Verification items for the finished model (mm, model axes). A direction names the side the tool comes from. Coordinates: 2 decimals unless noted, no trailing zeros. Order: outer loops, then holes, each group sorted by start corner. A loop starts at its lowest first (then second) coordinate and runs counter-clockwise, first axis right, second up. Notation, with made-up numbers: M 34,34.5 L 57,34.5 A17 ccw 57,56.5 Z; hole C 19.25,35.5 d2. An arc over 180 degrees is marked long. Return JSON: item names as keys, results as strings.
```python
from build123d import *

# Parameters (mm, degrees)
SKETCH1_W               = 89.5
SKETCH1_H               = 45.5
BOSS_EXTRUDE1_DEPTH     = 1.9
FILLET1_R               = 0.5
FILLET2_R               = 0.5
CUT_EXTRUDE1_DEPTH      = 75.270166564
CUT_EXTRUDE1_DEPTH_BACK = 75.270166564
SKETCH2_W               = 72
SKETCH2_H               = 25


with BuildPart() as part:
    # Sketch1 → Boss-Extrude1 (new body)
    with BuildSketch(Plane.XY):
        with Locations((-22.362297468, -9.005112503)):
            Rectangle(SKETCH1_W, SKETCH1_H)
    extrude(amount=BOSS_EXTRUDE1_DEPTH)

    # Fillet1
    fillet1_edges = [part.edges().sort_by_distance(p)[0] for p in [
        (22.387702532, -9.005112503, 1.9),
        (-22.362297468, 13.744887497, 1.9),
        (-67.112297468, -9.005112503, 1.9),
        (-22.362297468, 13.744887497, 0),
        (22.387702532, -9.005112503, 0),
        (-67.112297468, -9.005112503, 0),
        (-67.112297468, 13.744887497, 0.95),
        (22.387702532, 13.744887497, 0.95),
        (22.387702532, -31.755112503, 0.95),
        (-67.112297468, -31.755112503, 0.95),
    ]]
    fillet(fillet1_edges, radius=FILLET1_R)

    # Fillet2
    # the kernel refuses this fillet: 0.5 mm, written as the material it takes off along each edge
    with BuildSketch(Plane(origin=(-66.612297468, -31.255112503, 1.4), x_dir=(0, -1, 0), z_dir=(0, 0, 1))) as fillet2_piece_1_section:
        Polygon((0, 0), (FILLET2_R, 0), (FILLET2_R, -FILLET2_R), (0, -FILLET2_R), align=None)
    fillet2_piece_1 = extrude(amount=FILLET2_R, mode=Mode.PRIVATE)
    fillet2_piece_1 = fillet2_piece_1 - Plane(origin=(-66.612297468, -31.255112503, 1.4), x_dir=(0.7071067811865475, 0.7071067811865477, 0), z_dir=(0, 0, 1)) * Sphere(FILLET2_R, mode=Mode.PRIVATE)
    add(fillet2_piece_1, mode=Mode.SUBTRACT)
    with BuildSketch(Plane(origin=(-66.612297468, -31.255112503, 0.5), x_dir=(0, -1, 0), z_dir=(0, 0, -1))) as fillet2_piece_2_section:
        Polygon((0, 0), (FILLET2_R, 0), (FILLET2_R, FILLET2_R), (0, FILLET2_R), align=None)
    fillet2_piece_2 = extrude(amount=FILLET2_R, mode=Mode.PRIVATE)
    fillet2_piece_2 = fillet2_piece_2 - Plane(origin=(-66.612297468, -31.255112503, 0.5), x_dir=(0.7071067811865475, 0.7071067811865477, 0), z_dir=(0, 0, -1)) * Sphere(FILLET2_R, mode=Mode.PRIVATE)
    add(fillet2_piece_2, mode=Mode.SUBTRACT)
    with BuildSketch(Plane(origin=(21.887702532, -31.255112503, 1.4), x_dir=(0, -1, 0), z_dir=(0, 0, 1))) as fillet2_piece_3_section:
        Polygon((0, 0), (FILLET2_R, 0), (FILLET2_R, FILLET2_R), (0, FILLET2_R), align=None)
    fillet2_piece_3 = extrude(amount=FILLET2_R, mode=Mode.PRIVATE)
    fillet2_piece_3 = fillet2_piece_3 - Plane(origin=(21.887702532, -31.255112503, 1.4), x_dir=(-0.7071067811865476, 0.7071067811865474, 0), z_dir=(0, 0, 1)) * Sphere(FILLET2_R, mode=Mode.PRIVATE)
    add(fillet2_piece_3, mode=Mode.SUBTRACT)
    with BuildSketch(Plane(origin=(21.887702532, -31.255112503, 0.5), x_dir=(0, -1, 0), z_dir=(0, 0, -1))) as fillet2_piece_4_section:
        Polygon((0, 0), (FILLET2_R, 0), (FILLET2_R, -FILLET2_R), (0, -FILLET2_R), align=None)
    fillet2_piece_4 = extrude(amount=FILLET2_R, mode=Mode.PRIVATE)
    fillet2_piece_4 = fillet2_piece_4 - Plane(origin=(21.887702532, -31.255112503, 0.5), x_dir=(-0.7071067811865476, 0.7071067811865474, 0), z_dir=(0, 0, -1)) * Sphere(FILLET2_R, mode=Mode.PRIVATE)
    add(fillet2_piece_4, mode=Mode.SUBTRACT)
    with BuildSketch(Plane(origin=(21.887702532, -31.755112503, 0), x_dir=(0, 1, 0), z_dir=(-1, 0, 0))) as fillet2_piece_5:
        with BuildLine():
            CenterArc((FILLET2_R, -FILLET2_R), FILLET2_R, 90, 90)
            Line((0, -FILLET2_R), (0, 0))
            Line((0, 0), (FILLET2_R, 0))
        make_face()
    extrude(amount=88.5, mode=Mode.SUBTRACT)
    with BuildSketch(Plane(origin=(21.887702532, -31.755112503, 1.9), x_dir=(0, 1, 0), z_dir=(-1, 0, 0))) as fillet2_piece_6:
        with BuildLine():
            CenterArc((FILLET2_R, FILLET2_R), FILLET2_R, 180, 90)
            Line((0, FILLET2_R), (0, 0))
            Line((0, 0), (FILLET2_R, 0))
        make_face()
    extrude(amount=88.5, mode=Mode.SUBTRACT)

    # Sketch2 → Cut-Extrude1 (cut, two sides: drawn at the far end of the back side and taken through both)
    with BuildSketch(Plane.XY.offset(1.9).offset(-CUT_EXTRUDE1_DEPTH_BACK)):
        with Locations((-25.112297468, -11.755112503)):
            Rectangle(SKETCH2_W, SKETCH2_H)
    extrude(amount=CUT_EXTRUDE1_DEPTH + CUT_EXTRUDE1_DEPTH_BACK, mode=Mode.SUBTRACT)


solid = part.part
```
Q1. Draft check along X on faces 3 (the face through (-23, 1, 1.9)), 4 (the face through (-26, 0.745, 1)). Enter one of: pulls with the +X half, pulls with the -X half, needs draft (parallel to the pull), parting line crosses it, or undercut.
Values:
{"face 3": "needs draft", "face 4": "undercut"}
Q2. Cross-section at C-C, the plane z = 1.05. Record the boundary of the cut face in (x, y).
Values:
{"outline": "M -67.11,-31.26 A0.5 ccw -66.61,-31.76 L 21.89,-31.76 A0.5 ccw 22.39,-31.26 L 22.39,13.24 A0.5 ccw 21.89,13.74 L -66.61,13.74 A0.5 ccw -67.11,13.24 Z; hole M -61.11,-24.26 L 10.89,-24.26 L 10.89,0.74 L -61.11,0.74 Z"}
Q3. Go/stop test with a flat-tipped pin: pin 1 (0.6 mm diameter, centred on y = -13, z = 1.5, fed in from -X). Record where the tip stops, or that it passes through.
Values:
{"pin 1": "x = -67.11"}
Q4. Cross-section at A-A, the plane y = -3.5. Record the boundary of the cut face in (x, z).
Values:
{"outline": "M -67.11,0.5 A0.5 ccw -66.61,0 L -61.11,0 L -61.11,1.9 L -66.61,1.9 A0.5 ccw -67.11,1.4 Z; M 10.89,0 L 21.89,0 A0.5 ccw 22.39,0.5 L 22.39,1.4 A0.5 ccw 21.89,1.9 L 10.89,1.9 Z"}
Q5. Cross-section at B-B, the plane x = -7. Record the boundary of the cut face in (y, z).
Values:
{"outline": "M -31.76,0.5 A0.5 ccw -31.26,0 L -24.26,0 L -24.26,1.9 L -31.26,1.9 A0.5 ccw -31.76,1.4 Z; M 0.74,0 L 13.24,0 A0.5 ccw 13.74,0.5 L 13.74,1.4 A0.5 ccw 13.24,1.9 L 0.74,1.9 Z"}
Q6. Material ranges on line 1 along Y through (x, z) = (-20, 0.95); line 2 along X through (y, z) = (-2.5, 1.05); line 3 along Y through (x, z) = (-36, 0.4), recorded low to high.
Values:
{"line 1": "-31.76 to -24.26, 0.74 to 13.74", "line 2": "-67.11 to -61.11, 10.89 to 22.39", "line 3": "-31.75 to -24.26, 0.74 to 13.73"}
Q7. Tool access check on faces 1 (the face through (-23, 1, 0)), 2 (the face through (10.888, -12, 1)). Record the directions out of +Z, -Z, +X, -X, +Y, -Y that give a thin tool (end or side, any length) a straight path to the whole face; none if there is none.
Values:
{"face 1": "-Z, +X, -X, +Y, -Y", "face 2": "+Z, -Z"}
